from build123d import *

# Parameters (mm, degrees)
SKETCH035_R                               = 1.625
EXTRUDE011_DEPTH                          = 20
SKETCH020_W                               = 11
SKETCH020_H                               = 30
SKETCH020_R                               = 1.625
EXTRUDE004_DEPTH                          = 5
SKETCH022_AS_DRAWN_W                      = 72
SKETCH022_AS_DRAWN_H                      = 98
EXTRUDE006_DEPTH                          = 4.5
EXTRUDE006_ONTO_SKETCH022_ROLL_ANGLE      = 0
EXTRUDE006_ONTO_SKETCH022_PITCH_ANGLE     = 0
EXTRUDE006_ONTO_SKETCH022_PLACEMENT_ANGLE = 90.000003
SKETCH019_R                               = 1.125
SKETCH019_R_2                             = 1.625
EXTRUDE003_DEPTH                          = 5
SKETCH021_R                               = 1.125
EXTRUDE005_DEPTH                          = 5


with BuildPart() as basecuts001:
    # Sketch035 → Extrude011 (new body)
    with BuildSketch(Plane.XY):
        with Locations((-42, -332)):
            Circle(SKETCH035_R)
        with Locations((42, -332)):
            Circle(SKETCH035_R)
        with Locations((42, -272)):
            Circle(SKETCH035_R)
        with Locations((-42, -272)):
            Circle(SKETCH035_R)
    extrude(amount=EXTRUDE011_DEPTH)


with BuildPart() as basecuts001_1:
    # Extrude011 placement: moved
    add(basecuts001.part.moved(Location((0, 0, -329))))


with BuildPart() as gpshold:
    # Sketch020 → Extrude004 (new body)
    with BuildSketch(Plane.XY):
        with Locations((-13.5, -310)):
            Rectangle(SKETCH020_W, SKETCH020_H)
        with Locations((-13.45, -300.1)):
            Circle(SKETCH020_R, mode=Mode.SUBTRACT)
        with Locations((-13.45, -320.5)):
            Circle(SKETCH020_R, mode=Mode.SUBTRACT)
    extrude(amount=EXTRUDE004_DEPTH)


with BuildPart() as gpshold_1:
    # Extrude004 placement: moved
    add(gpshold.part.moved(Location((0, 0, -278))))


with BuildPart() as base:
    # Sketch022 as drawn → Extrude006 (new)
    with BuildSketch(Plane.XY):
        Rectangle(SKETCH022_AS_DRAWN_W, SKETCH022_AS_DRAWN_H)
    extrude(amount=EXTRUDE006_DEPTH)


with BuildPart() as base_1:
    # Extrude006 onto Sketch022 roll: moved
    add(base.part.rotate(Axis((0, 0, 0), (1, 0, 0)), EXTRUDE006_ONTO_SKETCH022_ROLL_ANGLE))


with BuildPart() as base_2:
    # Extrude006 onto Sketch022 pitch: moved
    add(base_1.part.rotate(Axis((0, 0, 0), (0, 1, 0)), EXTRUDE006_ONTO_SKETCH022_PITCH_ANGLE))


with BuildPart() as base_3:
    # Extrude006 onto Sketch022 placement: moved
    add(base_2.part.moved(Location((0, -302, -283.455178))).rotate(Axis((0, -302, -283.455178), (0, 0, 1)), EXTRUDE006_ONTO_SKETCH022_PLACEMENT_ANGLE))


with BuildPart() as base_4:
    # Extrude006 placement: moved
    add(base_3.part.moved(Location((0, 0, -44.75))))


with BuildPart() as obj1:
    # Sketch019 → Extrude003 (new body)
    with BuildSketch(Plane.XZ):
        Polygon((28, -324), (28, -316), (-8, -316), (-8, -278), (-19, -278), (-19, -316), (-34, -316), (-34, -324), align=None)
        with Locations((-29.8, -320.46)):
            Circle(SKETCH019_R, mode=Mode.SUBTRACT)
        with Locations((-13.58, -288.46)):
            Circle(SKETCH019_R, mode=Mode.SUBTRACT)
        with Locations((-0.15, -319.37)):
            Circle(SKETCH019_R_2, mode=Mode.SUBTRACT)
        with Locations((20.15, -319.37)):
            Circle(SKETCH019_R_2, mode=Mode.SUBTRACT)
    extrude(amount=EXTRUDE003_DEPTH)


with BuildPart() as obj1_1:
    # Extrude003 placement: moved
    add(obj1.part.moved(Location((0, -312, 0))))


with BuildPart() as base002:
    # Sketch021 (on Extrude) → Extrude005 (new body)
    with BuildSketch(Plane.XZ.offset(312)):
        Polygon((-25, -324), (-25, -316), (16.5, -316), (16.5, -278), (24.5, -278), (24.5, -324), align=None)
        with Locations((-20.4, -319.4)):
            Circle(SKETCH021_R, mode=Mode.SUBTRACT)
        with Locations((20.4, -282.6)):
            Circle(SKETCH021_R, mode=Mode.SUBTRACT)
    extrude(amount=EXTRUDE005_DEPTH)


with BuildPart() as base002_1:
    # Extrude005 placement: moved
    add(base002.part.moved(Location((0, 32, 0))))

    # Fusion038: union gpsHold, base, obj1
    add(gpshold_1.part)
    add(base_4.part)
    add(obj1_1.part)

    # Cut019: cut baseCuts001
    add(basecuts001_1.part, mode=Mode.SUBTRACT)


solid = base002_1.part
Here's how the part is built. I have some questions about the finished solid (model axes, mm). A direction names the side the tool comes from. Coordinates: 2 decimals unless noted, no trailing zeros. Order: outer loops, then holes, each group sorted by start corner. A loop starts at its lowest first (then second) coordinate and runs counter-clockwise, first axis right, second up. Notation, with made-up numbers: (16.25, 11) - (69.25, 11) arc R26 ccw to (69.25, 45) - close; hole circle Ø5 at (80, -10.5). An arc over 180 degrees is marked (long way). Use CSV: the item, a comma, the result in double quotes. Start each with the question number.
1. Suppose I cut it at C-C on x = -0.15. List the corners of the cut face in (y, z) for me (3 decimals).
2. I'm going to push flat-ended pins straight in: pin 1 (1.5 mm diameter, centred on y = -313.5, z = -318.5, fed in from +X); pin 2 (4 mm diameter, centred on x = -13.45, y = -320.5, fed in from +Z); pin 3 (1.5 mm diameter, centred on x = -10.5, y = -282.5, fed in from +Z); pin 4 (12 mm diameter, centred on x = 23, y = -303, fed in from +Z). Where does each tip first touch, or does it pass through?
3. Suppose I cut it at A-A on x = -42. List the corners of the cut face in (y, z) for me (3 decimals), then the cut area to 3 significant figures.
4. Suppose I cut it at D-D on z = -282.6. List the corners of the cut face in (x, y) for me (3 decimals).
5. Suppose I cut it at B-B on z = -304.5. List the corners of the cut face in (x, y) for me.
6. For faces 4 (the face through (-34, -314, -320)), 5 (the face through (-13.66, -318.89, -275.54)), 6 (the face through (-0.502, -314.465, -320.956)), which set-ups out of +Z, -Z, +X, -X, +Y, -Y let a thin tool reach every point of the face, with its end or its side?
7. If we mould it in two halves opening along Y, with no side actions, what happens to faces 1 (the face through (1, -338, -326)), 2 (the face through (41.79, -330.39, -325.99)), 3 (the face through (-1, -303, -328.205))? For each: +Y half, -Y half, draft (parallel to the pull), parting line (faces both ways), or undercut.
8. Please list where these lines run through material, in increasing order: line 1 (X direction, y = -272, z = -326) (3 decimals); line 2 (Y direction, x = -42, z = -326.6) (3 decimals); line 3 (X direction, y = -315.55, z = -288.46) (3 decimals). Write a range as from..to.
Output:
1,outline,"(-338, -328.205) - (-266, -328.205) - (-266, -323.705) - (-280, -323.705) - (-280, -316) - (-285, -316) - (-285, -323.705) - (-312, -323.705) - (-312, -320.995) - (-317, -320.995) - (-317, -323.705) - (-338, -323.705) - close; (-317, -317.745) - (-312, -317.745) - (-312, -316) - (-317, -316) - close"
2,pin 1,"stops at x = 28"
2,pin 2,"stops at z = -273"
2,pin 3,"stops at z = -316"
2,pin 4,"stops at z = -323.71"
3,outline,"(-338, -328.205) - (-333.625, -328.205) - (-333.625, -323.705) - (-338, -323.705) - close; (-330.375, -328.205) - (-273.625, -328.205) - (-273.625, -323.705) - (-330.375, -323.705) - close; (-270.375, -328.205) - (-266, -328.205) - (-266, -323.705) - (-270.375, -323.705) - close"
3,area,"295 mm2"
4,outline,"(-19, -317) - (-8, -317) - (-8, -312) - (-19, -312) - close; (16.5, -285) - (19.275, -285) - (19.275, -280) - (16.5, -280) - close; (21.525, -285) - (24.5, -285) - (24.5, -280) - (21.525, -280) - close"
5,outline,"(-19, -317) - (-8, -317) - (-8, -312) - (-19, -312) - close; (16.5, -285) - (24.5, -285) - (24.5, -280) - (16.5, -280) - close"
6,face 4,"+Z, -X, +Y, -Y"
6,face 5,"+Z"
6,face 6,"-Y"
7,face 1,"-Y half"
7,face 2,"undercut"
7,face 3,"draft"
8,line 1,"x = -49..-43.625, -40.375..40.375, 43.625..49"
8,line 2,"y = -338..-333.625, -330.375..-273.625, -270.375..-266"
8,line 3,"x = -19..-14.705, -12.455..-8"
